Can you work these out from the model? Positions are in its coordinate system, mm. A direction names the side the tool comes from. Give positions to 0.01 mm unless a question says otherwise; leave off trailing zeros. Loops run counter-clockwise (first coordinate to the right, second up) from the corner with the lowest first, then second, coordinate; pieces in that order, holes last. Notation, with made-up numbers: M 35,-11 L 73,-11 A20 ccw 73,-7 Z; hole C 57,41.25 d6. An arc over 180 degrees is marked long. Use CSV: the item, a comma, the result in double quotes.
from build123d import *

# Parameters (mm, degrees)
F0_W     = 21
F0_H     = 35
F0_W_2   = 19
F0_H_2   = 24.2712582345
F1_DEPTH = 9
F2_DEPTH = 1.5
F3_DEPTH = 5
F0_W_3   = 0.7944880121
F0_H_3   = 3.5
F4_DEPTH = 8


# Not quite as in the source:
# - a feature names something its author has since deleted; it is built from what else it names


with BuildPart() as f1:
    # F0 (on Front) → F1 (new body)
    with BuildSketch(Plane.XZ):
        Rectangle(F0_W, F0_H)
        Polygon((-9.3731830162, -10.6923110513), (-9.3731830162, -8.5423110513), (9.3731830162, -8.5423110513), (9.3731830162, -10.6923110513), (10.1676710284, -10.6923110513), (10.1676710284, -14.1923110513), (9.3731830162, -14.1923110513), (9.3731830162, -16.3423110513), (-9.3731830162, -16.3423110513), (-9.3731830162, -14.1923110513), (-10.1676710284, -14.1923110513), (-10.1676710284, -10.6923110513), align=None, mode=Mode.SUBTRACT)
        with Locations((0, 4.7412435117)):
            Rectangle(F0_W_2, F0_H_2, mode=Mode.SUBTRACT)
    extrude(amount=F1_DEPTH)

    # F0 (on Front) → F2 (join)
    with BuildSketch(Plane.XZ):
        with Locations((0, 4.7412435117)):
            Rectangle(F0_W_2, F0_H_2)
    extrude(amount=F2_DEPTH)

    # F0 (on Front) → F3 (join)
    with BuildSketch(Plane.XZ):
        Polygon((9.3731830162, -8.5423110513), (-9.3731830162, -8.5423110513), (-9.3731830162, -10.6923110513), (-9.3731830162, -14.1923110513), (-9.3731830162, -16.3423110513), (9.3731830162, -16.3423110513), (9.3731830162, -14.1923110513), (9.3731830162, -10.6923110513), align=None)
    extrude(amount=F3_DEPTH)

    # F0 (on Front) → F4 (join)
    with BuildSketch(Plane.XZ):
        with Locations((9.7704270223, -12.4423110513)):
            Rectangle(F0_W_3, F0_H_3)
        with Locations((-9.7704270223, -12.4423110513)):
            Rectangle(F0_W_3, F0_H_3)
    extrude(amount=F4_DEPTH)


solid = f1.part
Q1. Please list where these lines run through material, in increasing order: L1, parallel to Z at x = 5.5, y = -7.25; L2, parallel to X at y = -4, z = 4; L3, parallel to Z at x = 1.75, y = -4.75. Write a range as from..to.
Model answer:
L1,"-17.5..-16.34, -8.54..-7.39, 16.88..17.5"
L2,"-10.5..-9.5, 9.5..10.5"
L3,"-17.5..-7.39, 16.88..17.5"
Q2. I want a section at D-D, the plane z = -15. Please give me the cut outline in (x, y).
Model answer:
outline,"M -10.5,-9 L -9.37,-9 L -9.37,-5 L 9.37,-5 L 9.37,-9 L 10.5,-9 L 10.5,0 L -10.5,0 Z"
Q3. I want a section at C-C, the plane y = -2.75. Please give me the cut outline in (x, z), then the cut area to 3 significant figures.
Model answer:
outline,"M -10.5,-17.5 L 10.5,-17.5 L 10.5,17.5 L -10.5,17.5 Z; hole M -9.5,-7.39 L 9.5,-7.39 L 9.5,16.88 L -9.5,16.88 Z"
area,"274 mm2"
Q4. If we mould it in two halves opening along X, with no side actions, what happens to faces 3 (the flat face through (10.5, -4, 0)), 4 (the flat face through (0, -1.5, 5)), 5 (the flat face through (0, -9, -8))? For each: released by +X, released by -X, zero draft, split by the parting line, or undercut.
Model answer:
face 3,"released by +X"
face 4,"undercut"
face 5,"zero draft"
Q5. For faces 1 (the flat face through (-10.168, -8.5, -12.5)), 2 (the flat face through (-10.5, -4, 0)), which set-ups out of +Z, -Z, +X, -X, +Y, -Y let a thin tool reach every point of the face, with its end or its side?
Model answer:
face 1,"-Y"
face 2,"+Z, -Z, -X, +Y, -Y"
Q6. I want a section at A-A, the plane x = 3.5. Please give me the cut outline in (y, z), then the cut area to 3 significant figures.
Model answer:
outline,"M -9,-17.5 L 0,-17.5 L 0,17.5 L -9,17.5 L -9,16.88 L -1.5,16.88 L -1.5,-7.39 L -9,-7.39 L -9,-8.54 L -5,-8.54 L -5,-16.34 L -9,-16.34 Z"
area,"102 mm2"
Q7. I want a section at B-B, the plane y = -7. Please give me the cut outline in (x, z), then the cut area to 3 significant figures.
Model answer:
outline,"M -10.5,-17.5 L 10.5,-17.5 L 10.5,17.5 L -10.5,17.5 Z; hole M -9.5,-7.39 L 9.5,-7.39 L 9.5,16.88 L -9.5,16.88 Z; hole M -9.37,-16.34 L 9.37,-16.34 L 9.37,-8.54 L -9.37,-8.54 Z"
area,"128 mm2"
